from build123d import *

# Parameters (mm, degrees)
SKETCH1_R          = 2.413
EXTRUDE1_DEPTH     = 82.55
CHAMFER3_SIZE      = 0.5953125
SKETCH6_R          = 3.96875
EXTRUDE2_DEPTH     = 4.826
CUT_EXTRUDE1_DEPTH = 2.9765625
CHAMFER1_SIZE      = 0.396875
CHAMFER2_SIZE      = 0.1984375


with BuildPart() as part:
    # Sketch1 → Extrude1 (new body)
    with BuildSketch(Plane.XY):
        Circle(SKETCH1_R)
    extrude(amount=-EXTRUDE1_DEPTH)

    # Chamfer3
    chamfer3_edges = [part.edges().sort_by_distance(p)[0] for p in [
        (-2.413, 0, 0),
    ]]
    chamfer(chamfer3_edges, length=CHAMFER3_SIZE)

    # Sketch6 → Extrude2 (add)
    with BuildSketch(Plane(origin=(0, 0, -82.55), x_dir=(-1, 0, 0), z_dir=(0, 0, -1))):
        Circle(SKETCH6_R)
    extrude(amount=EXTRUDE2_DEPTH)

    # Sketch7 → Cut-Extrude1 (cut)
    with BuildSketch(Plane(origin=(0, 0, -87.376), x_dir=(-1, 0, 0), z_dir=(0, 0, -1))):
        Polygon((0, 2.291358881), (-1.984375, 1.14567944), (-1.984375, -1.14567944), (0, -2.291358881), (1.984375, -1.14567944), (1.984375, 1.14567944), align=None)
    extrude(amount=-CUT_EXTRUDE1_DEPTH, mode=Mode.SUBTRACT)

    # Cut-Extrude2 cone 1 section (through the dimple's axis) → Cut-Extrude2 (revolve, cut)
    with BuildSketch(Plane(origin=(0, 0, -87.376), x_dir=(0, 1, 0), z_dir=(1, 0, 0))):
        Polygon((0, 0), (2.291358881, 0), (0, 2.291358881), align=None)
    revolve(axis=Axis((0, 0, -87.376), (0, 0, 1)), mode=Mode.SUBTRACT)

    # Chamfer1
    chamfer1_edges = [part.edges().sort_by_distance(p)[0] for p in [
        (3.96875, 0, -87.376),
    ]]
    chamfer(chamfer1_edges, length=CHAMFER1_SIZE)

    # Chamfer2
    chamfer2_edges = [part.edges().sort_by_distance(p)[0] for p in [
        (3.96875, 0, -82.55),
    ]]
    chamfer(chamfer2_edges, length=CHAMFER2_SIZE)


solid = part.part
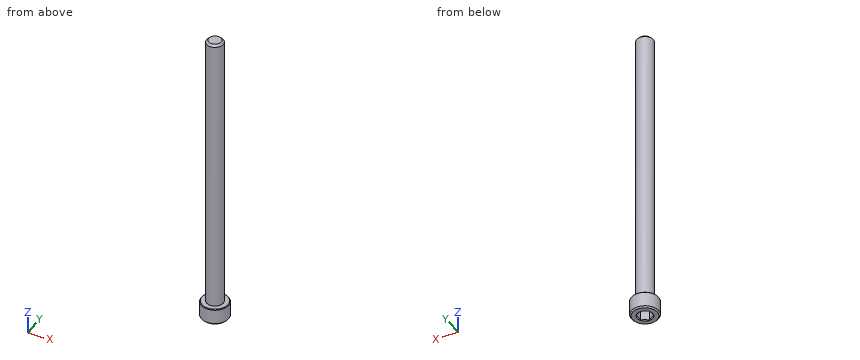
Work out the finished part from the listing and answer in its coordinate system (mm). Give positions to 0.01 mm unless a question says otherwise; leave off trailing zeros. Write each loop counter-clockwise with the first axis right and the second up, starting at its lowest first coordinate (ties: lowest second). Pieces come first, ordered by that corner, then holes.
Q1. Given pin 1 (1.8 mm diameter, centred on y = -0.5, z = -85, fed in from -X); pin 2 (1.5 mm diameter, centred on x = 1, z = -45.5, fed in from +Y); pin 3 (0.7 mm diameter, centred on y = 0.5, z = -86.5, fed in from +X); pin 4 (2 mm diameter, centred on x = 0.5, y = -0.5, fed in from -Z), each flat-ended and moving along its own axis, determine where each tip first touches the part or whether it passes through.
Answer:
pin 1: stops at x = -3.97
pin 2: stops at y = 2.4
pin 3: stops at x = 3.97
pin 4: stops at z = -84.4
Q2. The part is cut by section A-A on y = 0. Give the vertices of the cut face in (x, z).
Answer:
outline: (-3.97, -86.98) - (-3.57, -87.38) - (-2.29, -87.38) - (-1.98, -87.07) - (-1.98, -84.4) - (1.98, -84.4) - (1.98, -87.07) - (2.29, -87.38) - (3.57, -87.38) - (3.97, -86.98) - (3.97, -82.75) - (3.77, -82.55) - (2.41, -82.55) - (2.41, -0.6) - (1.82, 0) - (-1.82, 0) - (-2.41, -0.6) - (-2.41, -82.55) - (-3.77, -82.55) - (-3.97, -82.75) - close
Q3. The part is cut by section B-B on z = -25. Give the vertices of the cut face in (x, y), and give its area (3 significant figures).
Answer:
outline: circle Ø4.83 at (0, 0)
area: 18.3 mm2
Q4. Straight lines are drawn through the part: L1, parallel to Z at x = -0.75, y = 3; L2, parallel to Y at x = 0, z = -59; L3, parallel to Z at x = -1, y = -1.5. For each, find the intervals that lie inside material, in ascending order.
Answer:
L1: z = -87.38 to -82.55
L2: y = -2.41 to 2.41
L3: z = -84.4 to 0
